Verification items for the finished model (mm, model axes). Face numbers are marked on the shaded views. A direction names the side the tool comes from. Coordinates: 2 decimals unless noted, no trailing zeros. Order: outer loops, then holes, each group sorted by start corner. A loop starts at its lowest first (then second) coordinate and runs counter-clockwise, first axis right, second up. Notation, with made-up numbers: (13, -28.75) -> (27, -28.75) arc R28 ccw to (27, 4.25) -> close; hole circle Ø5 at (56, 79). An arc over 180 degrees is marked (long way). Answer as CSV lines item,"result".
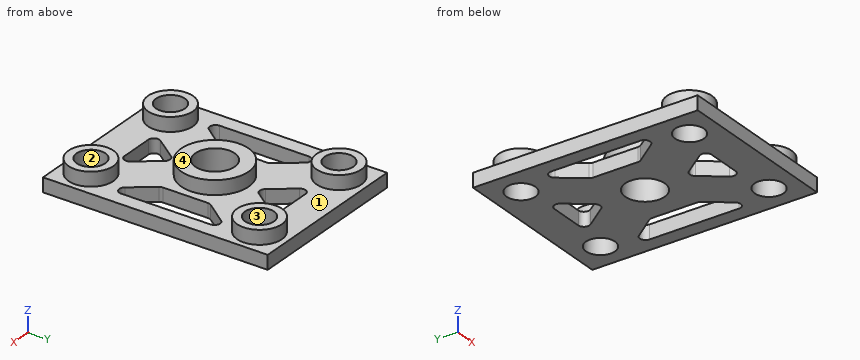
```python
from build123d import *

# Parameters (mm, degrees)
SKETCH1_W                           = 38.1
SKETCH1_H                           = 50.8
SKETCH1_R                           = 3.2639
SKETCH1_R_2                         = 4.445
BASE_EXTRUDE_DEPTH                  = 3.175
SKETCH2_R                           = 7.62
SKETCH2_R_2                         = 4.445
SKETCH2_R_3                         = 5.08
SKETCH2_R_4                         = 3.2639
RAISER_DEPTH                        = 3.175
WEIGHT_REDUCTION_SCREW_ACCESS_DEPTH = 4.175


with BuildPart() as part:
    # Sketch1 → Base Extrude (new body)
    with BuildSketch(Plane.XY):
        with Locations((19.05, -25.4)):
            Rectangle(SKETCH1_W, SKETCH1_H)
        with Locations((6.35, -6.35)):
            Circle(SKETCH1_R, mode=Mode.SUBTRACT)
        with Locations((6.35, -44.45)):
            Circle(SKETCH1_R, mode=Mode.SUBTRACT)
        with Locations((31.75, -44.45)):
            Circle(SKETCH1_R, mode=Mode.SUBTRACT)
        with Locations((31.75, -6.35)):
            Circle(SKETCH1_R, mode=Mode.SUBTRACT)
        with Locations((19.05, -25.4)):
            Circle(SKETCH1_R_2, mode=Mode.SUBTRACT)
    extrude(amount=BASE_EXTRUDE_DEPTH)

    # Sketch2 → Raiser (add)
    with BuildSketch(Plane.XY.offset(3.175)):
        with Locations((19.05, -25.4)):
            Circle(SKETCH2_R)
        with Locations((19.05, -25.4)):
            Circle(SKETCH2_R_2, mode=Mode.SUBTRACT)
        with Locations((6.35, -6.35)):
            Circle(SKETCH2_R_3)
        with Locations((6.35, -6.35)):
            Circle(SKETCH2_R_4, mode=Mode.SUBTRACT)
        with Locations((31.75, -6.35)):
            Circle(SKETCH2_R_3)
        with Locations((31.75, -6.35)):
            Circle(SKETCH2_R_4, mode=Mode.SUBTRACT)
        with Locations((6.35, -44.45)):
            Circle(SKETCH2_R_3)
        with Locations((6.35, -44.45)):
            Circle(SKETCH2_R_4, mode=Mode.SUBTRACT)
        with Locations((31.75, -44.45)):
            Circle(SKETCH2_R_3)
        with Locations((31.75, -44.45)):
            Circle(SKETCH2_R_4, mode=Mode.SUBTRACT)
    extrude(amount=RAISER_DEPTH)

    # Sketch3 → Weight Reduction - screw access (cut, through all)
    with BuildSketch(Plane.XY.offset(3.175)):
        with BuildLine():
            Line((3.302, -15.289677034), (3.302, -35.510322966))
            ThreePointArc((3.302, -35.510322966), (4.181713329, -36.730860012), (5.617806221, -36.282258372))
            Line((5.617806221, -36.282258372), (9.394688198, -31.246415736))
            ThreePointArc((9.394688198, -31.246415736), (9.585978035, -30.881326012), (9.652, -30.47448033))
            Line((9.652, -30.47448033), (9.652, -20.32551967))
            ThreePointArc((9.652, -20.32551967), (9.585978035, -19.918673988), (9.394688198, -19.553584264))
            Line((9.394688198, -19.553584264), (5.617806221, -14.517741628))
            ThreePointArc((5.617806221, -14.517741628), (4.181713329, -14.069139988), (3.302, -15.289677034))
        make_face()
        with BuildLine():
            Line((15.24, -7.62), (22.86, -7.62))
            ThreePointArc((22.86, -7.62), (23.993921047, -8.318053273), (23.881326665, -9.644845576))
            Line((23.881326665, -9.644845576), (20.126783029, -14.724845576))
            ThreePointArc((20.126783029, -14.724845576), (19.677403092, -15.103921047), (19.105456364, -15.24))
            Line((19.105456364, -15.24), (19.016881977, -15.24))
            ThreePointArc((19.016881977, -15.24), (18.448920711, -15.105922533), (18.000881977, -14.732))
            Line((18.000881977, -14.732), (14.210752791, -9.678494418))
            ThreePointArc((14.210752791, -9.678494418), (14.089266637, -8.33119233), (15.24, -7.62))
        make_face()
        with BuildLine():
            Line((14.218673335, -41.155154424), (17.973216971, -36.075154424))
            ThreePointArc((17.973216971, -36.075154424), (18.422596908, -35.696078953), (18.994543636, -35.56))
            Line((18.994543636, -35.56), (19.083118023, -35.56))
            ThreePointArc((19.083118023, -35.56), (19.651079289, -35.694077467), (20.099118023, -36.068))
            Line((20.099118023, -36.068), (23.889247209, -41.121505582))
            ThreePointArc((23.889247209, -41.121505582), (24.010733363, -42.46880767), (22.86, -43.18))
            Line((22.86, -43.18), (15.24, -43.18))
            ThreePointArc((15.24, -43.18), (14.106078953, -42.481946727), (14.218673335, -41.155154424))
        make_face()
        with BuildLine():
            Line((28.705311802, -31.246415736), (32.482193779, -36.282258372))
            ThreePointArc((32.482193779, -36.282258372), (33.918286671, -36.730860012), (34.798, -35.510322966))
            Line((34.798, -35.510322966), (34.798, -15.289677034))
            ThreePointArc((34.798, -15.289677034), (33.918286671, -14.069139988), (32.482193779, -14.517741628))
            Line((32.482193779, -14.517741628), (28.705311802, -19.553584264))
            ThreePointArc((28.705311802, -19.553584264), (28.514021965, -19.918673988), (28.448, -20.32551967))
            Line((28.448, -20.32551967), (28.448, -30.47448033))
            ThreePointArc((28.448, -30.47448033), (28.514021965, -30.881326012), (28.705311802, -31.246415736))
        make_face()
    extrude(amount=-WEIGHT_REDUCTION_SCREW_ACCESS_DEPTH, mode=Mode.SUBTRACT)


solid = part.part
```
Item 1: Thickness scan on line 1 (Y direction, x = 31.75, z = 4.5); line 2 (Y direction, x = 19.05, z = 4.5) (3 decimals); line 3 (Y direction, x = 6.35, z = 2). Record the ranges inside material, lowest first.
Answer list:
line 1,"-49.53 to -47.71, -41.19 to -39.37, -11.43 to -9.61, -3.09 to -1.27"
line 2,"-33.02 to -29.845, -20.955 to -17.78"
line 3,"-50.8 to -47.71, -41.19 to -35.31, -15.49 to -9.61, -3.09 to 0"
Item 2: Tool access check on the marked faces 1 and 2. Record the directions out of +Z, -Z, +X, -X, +Y, -Y that give a thin tool (end or side, any length) a straight path to the whole face; none if there is none.
Answer list:
face 1,"+Z"
face 2,"+Z, -Z"
Item 3: Section check C-C, the plane y = -25.4. Record the boundary of the cut face in (x, z) (3 decimals), plus the area to 3 significant figures.
Answer list:
outline,"(0, 0) -> (3.302, 0) -> (3.302, 3.175) -> (0, 3.175) -> close; (9.652, 0) -> (14.605, 0) -> (14.605, 6.35) -> (11.43, 6.35) -> (11.43, 3.175) -> (9.652, 3.175) -> close; (23.495, 0) -> (28.448, 0) -> (28.448, 3.175) -> (26.67, 3.175) -> (26.67, 6.35) -> (23.495, 6.35) -> close; (34.798, 0) -> (38.1, 0) -> (38.1, 3.175) -> (34.798, 3.175) -> close"
area,"72.6 mm2"
Item 4: Section check D-D, the plane x = 8. Record the boundary of the cut face in (y, z) (3 decimals).
Answer list:
outline,"(-50.8, 0) -> (-47.266, 0) -> (-47.266, 6.35) -> (-49.255, 6.35) -> (-49.255, 3.175) -> (-50.8, 3.175) -> close; (-41.634, 0) -> (-33.106, 0) -> (-33.106, 3.175) -> (-39.645, 3.175) -> (-39.645, 6.35) -> (-41.634, 6.35) -> close; (-17.694, 0) -> (-9.166, 0) -> (-9.166, 6.35) -> (-11.155, 6.35) -> (-11.155, 3.175) -> (-17.694, 3.175) -> close; (-3.534, 0) -> (0, 0) -> (0, 3.175) -> (-1.545, 3.175) -> (-1.545, 6.35) -> (-3.534, 6.35) -> close"
Item 5: Depth check by flat-ended pin: pin 1 Ø5 at (x, y) = (34, -6) entering from -Z; pin 2 Ø2 at (x, z) = (32.5, 5) entering from -Y. Enter the tip coordinate at first touch or a pass-through.
Answer list:
pin 1,"z = 0"
pin 2,"y = -49.53"
Item 6: Section check B-B, the plane y = -44.45. Record the boundary of the cut face in (x, z) (3 decimals), plus the area to 3 significant figures.
Answer list:
outline,"(0, 0) -> (3.086, 0) -> (3.086, 6.35) -> (1.27, 6.35) -> (1.27, 3.175) -> (0, 3.175) -> close; (9.614, 0) -> (28.486, 0) -> (28.486, 6.35) -> (26.67, 6.35) -> (26.67, 3.175) -> (11.43, 3.175) -> (11.43, 6.35) -> (9.614, 6.35) -> close; (35.014, 0) -> (38.1, 0) -> (38.1, 3.175) -> (36.83, 3.175) -> (36.83, 6.35) -> (35.014, 6.35) -> close"
area,"103 mm2"
Item 7: Release check for a two-part mould opening along X. For the marked faces 3 and 4 record: +X half, -X half, draft (parallel to the pull), parting line (faces both ways), or undercut.
Answer list:
face 3,"undercut"
face 4,"draft"
Item 8: Section check A-A, the plane z = 5.75. Count the separate pieces of the cut face and the enclosed holes in it, plus the area to 3 significant figures.
Answer list:
separate pieces,"5"
enclosed holes,"5"
area,"311 mm2"
